For this review, take the finished solid that the model builds, in its own axes (mm). A direction names the side the tool comes from. Give positions to 0.01 mm unless a question says otherwise; leave off trailing zeros. Order: outer loops, then holes, each group sorted by start corner. A loop starts at its lowest first (then second) coordinate and runs counter-clockwise, first axis right, second up.
Autodesk Inventor part; units mm, degrees
ref_plane "YZ Plane" through (0, 0, 0) normal (1, 0, 0) x (0, 1, 0)
ref_plane "XZ Plane" through (0, 0, 0) normal (0, 1, 0) x (-1, 0, 0)
ref_plane "XY Plane" through (0, 0, 0) normal (0, 0, 1) x (1, 0, 0)
sketch "Skizze1" plane through (0, 0, 0) normal (0, 1, 0) x (-1, 0, 0)
  line L0 (0, 0) -> (0, -100) construction
  line L1 (0, 0) -> (11, 0)
  arc A0 (14, -1) -> (11, 0) centre (11, -5) ccw
  line L2 (14, -1) -> (14, -2)
  line L3 (14, -2) -> (12.5, -2)
  line L4 (12.5, -2) -> (12.5, -14)
  arc A1 (11, -18) -> (12.5, -14) centre (6.4167, -14) ccw
  line L5 (11, -18) -> (9.25, -18)
  line L6 (9.25, -18) -> (9.25, -25.5)
  line L7 (9.25, -25.5) -> (0, -25.5)
  line L8 (0, 0) -> (0, -25.5)
  point P0 (13.25, -2)
  dimension "d0" = 100
  dimension "d1" = 25
  dimension "d2" = 28
  dimension "d3" = 2
  dimension "d4" = 1
  dimension "d5" = 3
  dimension "d6" = 12
  dimension "d7" = 4
  dimension "d8" = 22
  dimension "d9" = 18.5
  dimension "d10" = 7.5
revolve "Umdrehung1" add sketch "Skizze1" angle 360 about axis through (0, 0, 0) along (0, 0, -1)
thread "Gewinde1"
sketch "Skizze2" plane through (0, 0, -25.5) normal (0, 0, -1) x (-1, 0, 0)
  circle A0 centre (0, 0) radius 9.25
  line L0 (5, 7.7822) -> (-5, 7.7822)
  line L1 (-5, 7.7822) -> (-5, -7.7822)
  line L2 (-5, -7.7822) -> (5, -7.7822)
  line L3 (5, -7.7822) -> (5, 7.7822)
  dimension "d14" = 10
extrude "Extrusion1" cut sketch "Skizze2" against normal up to surface (7.5 mm away) contours A0 L3 | L1 A0
sketch "Skizze3" plane through (0, 0, -25.5) normal (0, 0, -1) x (-1, 0, 0)
  line L0 (3.5, 7) -> (3, 7)
  line L1 (3, 7) -> (3, 5)
  line L2 (3, 5) -> (3.5, 5)
  line L3 (3.5, 5) -> (3.5, 7)
  point P0 (0, 0)
  point P1 (3, 6)
  dimension "d17" = 0.5
  dimension "d18" = 2
  dimension "d19" = 5
  dimension "d20" = 3
extrude "Extrusion2" add sketch "Skizze3" along normal blind 6
pattern_linear "Rechteckige Anordnung1" count 3 spacing 3 along (1, 0, 0) of "Extrusion2"
properties part number "Druckknopf_Konsole_groß" material "Stahl, galvanisiert"
1) Tool access review of faces 1 (the face through (-12.932, -5.362, -1.507)), 2 (the face through (-3.5, 6, -28)), 3 (the face through (2.5, 6, -28)), 4 (the face through (5.3, 11.5, -2)), 5 (the face through (3, 6, -28)): name each direction out of +Z, -Z, +X, -X, +Y, -Y from which nothing blocks a thin tool from reaching the whole face with its end or side.
Answer sheet:
face 1: +Z, -Z
face 2: -Z, -X, +Y, -Y
face 3: -Z, +Y, -Y
face 4: -Z
face 5: -Z, +X, +Y, -Y
2) To check wall thickness, follow line 1 (Z direction, x = 3.25, y = 8); line 2 (X direction, y = -0.5, z = -23); line 3 (X direction, y = 0.25, z = -4). State the ranges of each line that lie inside material, in increasing order.
Answer sheet:
line 1: z = -25.5 to 0
line 2: x = -5 to 5
line 3: x = -12.5 to 12.5
3) We need section C-C on z = -15. Give the boundary of the cut face in (x, y).
Answer sheet:
outline: circle Ø24.83 at (0, 0)
4) We need section A-A on y = 0. Give the boundary of the cut face in (x, z).
Answer sheet:
outline: (-14, -2) - (-12.5, -2) - (-12.5, -14) arc R6.08 ccw to (-11, -18) - (-5, -18) - (-5, -25.5) - (5, -25.5) - (5, -18) - (11, -18) arc R6.08 ccw to (12.5, -14) - (12.5, -2) - (14, -2) - (14, -1) arc R5 ccw to (11, 0) - (-11, 0) arc R5 ccw to (-14, -1) - close
5) Clearance check with flat-ended pins moving along their axes: pin 1 (2 mm diameter, centred on x = -4.5, z = -7, fed in from +Y); pin 2 (0.6 mm diameter, centred on x = 0, z = -27.5, fed in from +Y); pin 3 (2 mm diameter, centred on x = -3, z = -18.5, fed in from +Y). State where each tip first meets the part, or that it passes through.
Answer sheet:
pin 1: stops at y = 12
pin 2: stops at y = 7
pin 3: stops at y = 11.03
6) We need section B-B on z = -3. Give the boundary of the cut face in (x, y), then the cut area to 3 significant figures.
Answer sheet:
outline: circle Ø25 at (0, 0)
area: 491 mm2
7) Draft analysis for pull direction Y (two halves, no side actions). For faces 6 (the face through (-0.07, 9.25, -21.8)), 7 (the face through (-3, 6, -28)), 8 (the face through (-11.923, 3.755, -8.084)), 9 (the face through (0.07, -9.25, -21.8)), state which applies: +Y half, -Y half, draft (parallel to the pull), parting line (faces both ways), or undercut.
Answer sheet:
face 6: +Y half
face 7: draft
face 8: parting line
face 9: -Y half
